from build123d import *

# Parameters (mm, degrees)
MODEL_R                 = 2.1
BOSS_EXTRU_1_DEPTH      = 8
ESQUISSE2_W             = 619.951628201
ESQUISSE2_H             = 4
ENL_V_MAT_EXTRU_1_DEPTH = 2
CHANFREIN1_SIZE         = 1
ENL_V_MAT_EXTRU_2_DEPTH = 55.986789313


with BuildPart() as part:
    # Model → Boss.-Extru.1 (new body)
    with BuildSketch(Plane.XY):
        with BuildLine():
            Line((5.807601336, 84.65), (5.807601336, 156.65))
            ThreePointArc((5.807601336, 156.65), (6.979174211, 159.478427125), (9.807601336, 160.65))
            Line((9.807601336, 160.65), (112.089987365, 160.65))
            ThreePointArc((112.089987365, 160.65), (114.746116476, 159.886151336), (116.590693318, 157.827991258))
            Line((116.590693318, 157.827991258), (125.144495245, 140.1520033))
            ThreePointArc((125.144495245, 140.1520033), (128.095818192, 136.858947175), (132.34562477, 135.636789313))
            Line((132.34562477, 135.636789313), (707.759229537, 135.636789313))
            ThreePointArc((707.759229537, 135.636789313), (713.416083787, 133.293643563), (715.759229537, 127.636789313))
            Line((715.759229537, 127.636789313), (715.759229537, 122.65))
            Line((715.759229537, 122.65), (625.759229537, 122.65))
            Line((625.759229537, 122.65), (625.759229537, 118.65))
            Line((625.759229537, 118.65), (715.759229537, 118.65))
            Line((715.759229537, 118.65), (715.759229537, 113.663210687))
            ThreePointArc((715.759229537, 113.663210687), (713.416083787, 108.006356437), (707.759229537, 105.663210687))
            Line((707.759229537, 105.663210687), (132.34562477, 105.663210687))
            ThreePointArc((132.34562477, 105.663210687), (128.095818192, 104.441052825), (125.144495245, 101.1479967))
            Line((125.144495245, 101.1479967), (116.590693318, 83.472008742))
            ThreePointArc((116.590693318, 83.472008742), (114.746116476, 81.413848664), (112.089987365, 80.65))
            Line((112.089987365, 80.65), (9.807601336, 80.65))
            ThreePointArc((9.807601336, 80.65), (6.979174211, 81.821572875), (5.807601336, 84.65))
        make_face()
        with Locations((702.759229537, 129.143394657)):
            Circle(MODEL_R, mode=Mode.SUBTRACT)
        with Locations((702.759229537, 112.156605343)):
            Circle(MODEL_R, mode=Mode.SUBTRACT)
        with Locations((47.853374331, 154.15)):
            Circle(MODEL_R, mode=Mode.SUBTRACT)
        with Locations((97.853374331, 154.15)):
            Circle(MODEL_R, mode=Mode.SUBTRACT)
        with Locations((22.853374331, 154.15)):
            Circle(MODEL_R, mode=Mode.SUBTRACT)
        with Locations((72.853374331, 154.15)):
            Circle(MODEL_R, mode=Mode.SUBTRACT)
        with Locations((47.853374331, 87.15)):
            Circle(MODEL_R, mode=Mode.SUBTRACT)
        with Locations((97.853374331, 87.15)):
            Circle(MODEL_R, mode=Mode.SUBTRACT)
        with Locations((22.853374331, 87.15)):
            Circle(MODEL_R, mode=Mode.SUBTRACT)
        with Locations((72.853374331, 87.15)):
            Circle(MODEL_R, mode=Mode.SUBTRACT)
        with BuildLine():
            Line((15.807601336, 84.988017314), (15.807601336, 102.988017314))
            ThreePointArc((15.807601336, 102.988017314), (14.807601336, 103.988017314), (13.807601336, 102.988017314))
            Line((13.807601336, 102.988017314), (13.807601336, 84.988017314))
            ThreePointArc((13.807601336, 84.988017314), (14.807601336, 83.988017314), (15.807601336, 84.988017314))
        make_face(mode=Mode.SUBTRACT)
        with BuildLine():
            Line((15.807601336, 156.311982686), (15.807601336, 138.311982686))
            ThreePointArc((15.807601336, 138.311982686), (14.807601336, 137.311982686), (13.807601336, 138.311982686))
            Line((13.807601336, 138.311982686), (13.807601336, 156.311982686))
            ThreePointArc((13.807601336, 156.311982686), (14.807601336, 157.311982686), (15.807601336, 156.311982686))
        make_face(mode=Mode.SUBTRACT)
    extrude(amount=BOSS_EXTRU_1_DEPTH)

    # Esquisse2 → Enlèv. mat.-Extru.1 (cut)
    with BuildSketch(Plane.XY.offset(8)):
        with Locations((315.783415436, 120.65)):
            Rectangle(ESQUISSE2_W, ESQUISSE2_H)
    extrude(amount=-ENL_V_MAT_EXTRU_1_DEPTH, mode=Mode.SUBTRACT)

    # Chanfrein1
    chanfrein1_edges = [part.edges().sort_by_distance(p)[0] for p in [
        (14.807601336, 103.988017314, 0),
        (13.807601336, 93.988017314, 0),
        (14.807601336, 83.988017314, 0),
        (15.807601336, 93.988017314, 0),
        (700.659229537, 129.143394657, 0),
        (700.659229537, 112.156605343, 0),
        (45.753374331, 154.15, 0),
        (95.753374331, 154.15, 0),
        (20.753374331, 154.15, 0),
        (70.753374331, 154.15, 0),
        (45.753374331, 87.15, 0),
        (95.753374331, 87.15, 0),
        (20.753374331, 87.15, 0),
        (70.753374331, 87.15, 0),
        (14.807601336, 157.311982686, 0),
        (13.807601336, 147.311982686, 0),
        (14.807601336, 137.311982686, 0),
        (15.807601336, 147.311982686, 0),
    ]]
    chamfer(chanfrein1_edges, length=CHANFREIN1_SIZE)

    # Esquisse3 → Enlèv. mat.-Extru.2 (cut, through all)
    with BuildSketch(Plane.XZ.offset(-105.663210687)):
        with BuildLine():
            Line((235.807601336, 8), (285.807601336, 8))
            ThreePointArc((285.807601336, 8), (260.807601336, 6.5), (235.807601336, 8))
        make_face()
        with BuildLine():
            Line((432.807601336, 8), (482.807601336, 8))
            ThreePointArc((482.807601336, 8), (457.807601336, 6.5), (432.807601336, 8))
        make_face()
    extrude(amount=-ENL_V_MAT_EXTRU_2_DEPTH, mode=Mode.SUBTRACT)


solid = part.part
Build history of the part. All positions in model axes, mm. Round coordinates to 2 decimals unless told otherwise and drop trailing zeros. Loops run counter-clockwise (first coordinate to the right, second up) from the corner with the lowest first, then second, coordinate; pieces in that order, holes last. Notation, with made-up numbers: (24.25, 65.5) -> (60.25, 65.5) arc R27 cw to (60.25, 81.5) -> close; hole circle Ø5 at (70, 84.25). An arc over 180 degrees is marked (long way). One line per item, written item: value. Start each with the question number.
Q1. Cut at A-A on x = 554.5. List the corners of the cut face in (y, z).
Q2. Two-plate mould, pull along X, no slides. Class faces 1 (the face through (97, 138, 8)), 2 (the face through (261.2, 129.1, 6.5)), 3 (the face through (458.2, 112.1, 6.5)): released by +X, released by -X, zero draft, split by the parting line, or undercut.
Q3. Probe line 1 along Y through (x, z) = (48, 6.75); line 2 along X through (y, z) = (87.5, 5); line 3 along Y through (x, z) = (626, 1.25). List the from-to ranges inside material, lowest first.
Q4. Drop flat-ended pins along their axis: pin 1 Ø6 at (x, y) = (243, 128) entering from +Z; pin 2 Ø2 at (y, z) = (120, 3.5) entering from +X; pin 3 Ø5 at (x, y) = (97.85, 154.15) entering from -Z. Give the stop position or say it passes through.
Q5. Cut at B-B on z = 4. Count the separate pieces of the cut face and the enclosed holes in it, plus the area to 3 significant figures.
Computed:
1. outline: (105.66, 0) -> (135.64, 0) -> (135.64, 8) -> (122.65, 8) -> (122.65, 6) -> (118.65, 6) -> (118.65, 8) -> (105.66, 8) -> close
2. face 1: zero draft
2. face 2: undercut
2. face 3: undercut
3. line 1: 80.65 to 85.06, 89.24 to 118.65, 122.65 to 152.06, 156.24 to 160.65
3. line 2: 5.81 to 13.81, 15.81 to 20.78, 24.92 to 45.78, 49.92 to 70.78, 74.92 to 95.78, 99.92 to 118.54
3. line 3: 105.66 to 118.65, 122.65 to 135.64
4. pin 1: z = 7.54
4. pin 2: x = 625.76
4. pin 3: z = 0.6
5. separate pieces: 1
5. enclosed holes: 12
5. area: 26,500 mm²
